from build123d import *

# Parameters (mm, degrees)
SKETCH_1_R          = 1.55
SKETCH_1_R_2        = 1.3
EXTRUDE_1_DEPTH     = 3
FILLET_1_R          = 1
SKETCH_2_W          = 7.568949752
SKETCH_2_H          = 24.928305666
CUT_EXTRUDE_1_DEPTH = 10


with BuildPart() as part:
    # 草图1 → 凸台-拉伸1 (new body)
    with BuildSketch(Plane(origin=(0, 0, 0), x_dir=(0, 0, -1), z_dir=(1, 0, 0))):
        with BuildLine():
            Line((-11, -27.75), (11, -27.75))
            Line((11, -27.75), (11, 19.65))
            Line((11, 19.65), (28.4, 19.65))
            Line((28.4, 19.65), (28.4, 25.85))
            ThreePointArc((28.4, 25.85), (29.45, 26.9), (30.5, 25.85))
            Line((30.5, 25.85), (43.6, 25.85))
            Line((43.6, 25.85), (43.6, 19.65))
            Line((43.6, 19.65), (45.6, 19.65))
            Line((45.6, 19.65), (45.6, 29.85))
            Line((45.6, 29.85), (19.913066695, 41.248539803))
            Line((19.913066695, 41.248539803), (-11, 27.75))
            Line((-11, 27.75), (-11, -27.75))
        make_face()
        with Locations((-8, -19.75)):
            Circle(SKETCH_1_R, mode=Mode.SUBTRACT)
        with Locations((0, -23.25)):
            Circle(SKETCH_1_R, mode=Mode.SUBTRACT)
        with Locations((0, -16.25)):
            Circle(SKETCH_1_R, mode=Mode.SUBTRACT)
        with Locations((8, -19.75)):
            Circle(SKETCH_1_R, mode=Mode.SUBTRACT)
        Polygon((5.344705464, -11.25), (-5.344705464, -11.25), (0, 0.202940281), align=None, mode=Mode.SUBTRACT)
        Polygon((-7, -7.702940281), (-7, 15.202940281), (-1.655294536, 3.75), align=None, mode=Mode.SUBTRACT)
        Polygon((7, 15.202940281), (7, -7.702940281), (1.655294536, 3.75), align=None, mode=Mode.SUBTRACT)
        with Locations((-6, 23.75)):
            Circle(SKETCH_1_R, mode=Mode.SUBTRACT)
        with BuildLine():
            Line((2, 16.7), (-2, 16.7))
            ThreePointArc((-2, 16.7), (-3.05, 15.65), (-4.1, 16.7))
            Line((-4.1, 16.7), (-4.1, 19.8))
            ThreePointArc((-4.1, 19.8), (-3.05, 20.85), (-2, 19.8))
            Line((-2, 19.8), (2, 19.8))
            ThreePointArc((2, 19.8), (3.05, 20.85), (4.1, 19.8))
            Line((4.1, 19.8), (4.1, 16.7))
            ThreePointArc((4.1, 16.7), (3.05, 15.65), (2, 16.7))
        make_face(mode=Mode.SUBTRACT)
        with Locations((6, 23.75)):
            Circle(SKETCH_1_R, mode=Mode.SUBTRACT)
        with Locations((15, 22.75)):
            Circle(SKETCH_1_R_2, mode=Mode.SUBTRACT)
        Polygon((11, 27.75), (-1.004338059, 27.75), (15.913066695, 35.137175905), (15.913066695, 27.75), align=None, mode=Mode.SUBTRACT)
        Polygon((23.913066695, 28.85), (23.913066695, 35.097405162), (37.991771729, 28.85), align=None, mode=Mode.SUBTRACT)
        with Locations((19.913066695, 36.248539803)):
            Circle(SKETCH_1_R_2, mode=Mode.SUBTRACT)
    extrude(amount=EXTRUDE_1_DEPTH)

    # 圆角1
    fillet_1_edges = [part.edges().sort_by_distance(p)[0] for p in [
        (1.5, 35.097405162, -23.913066695),
        (1.5, 28.85, -23.913066695),
        (1.5, 28.85, -37.991771729),
        (1.5, 35.137175905, -15.913066695),
        (1.5, 27.75, 1.004338059),
        (1.5, 27.75, -15.913066695),
        (1.5, 15.202940281, 7),
        (1.5, -7.702940281, 7),
        (1.5, 3.75, 1.655294536),
        (1.5, -7.702940281, -7),
        (1.5, 15.202940281, -7),
        (1.5, 3.75, -1.655294536),
        (1.5, -11.25, 5.344705464),
        (1.5, -11.25, -5.344705464),
        (1.5, 0.202940281, 0),
    ]]
    fillet(fillet_1_edges, radius=FILLET_1_R)

    # 草图2 → 切除-拉伸1 (cut)
    with BuildSketch(Plane(origin=(3, 0, 0), x_dir=(0, 0, -1), z_dir=(1, 0, 0))):
        with Locations((47.384474876, 32.114152833)):
            Rectangle(SKETCH_2_W, SKETCH_2_H)
    extrude(amount=-CUT_EXTRUDE_1_DEPTH, mode=Mode.SUBTRACT)


solid = part.part
Verification items for the finished model (mm, model axes). Coordinates: 2 decimals unless noted, no trailing zeros. Loops run counter-clockwise (first coordinate to the right, second up) from the corner with the lowest first, then second, coordinate; pieces in that order, holes last. Notation, with made-up numbers: (29, 63) -> (61, 63) arc R17 cw to (61, 70) -> close; hole circle Ø10 at (67.25, -8). An arc over 180 degrees is marked (long way). Answer as a JSON object with one key per item and string values. Group by question number.
Item 1: Sectioned sample at B-B on y = -19. Record the boundary of the cut face in (x, z), plus the area to 3 significant figures.
Item 2: Scan lines: probe 1 along Z at (x, y) = (2.7, 30); probe 2 along Y at (x, z) = (1.65, -5.5); probe 3 along Z at (x, y) = (1.4, 0.5). Record each from-to range of solid material in increasing order.
Item 3: Sectioned sample at A-A on z = 3.05. Record the boundary of the cut face in (x, y).
Item 4: Mould release check, pull along Z, two halves, no side actions. Record for faces 1 (the cylindrical face through (1.48, 20.85, 3.07)), 2 (the flat face through (1, 0, 11)): +Z half, -Z half, draft (parallel to the pull), parting line (faces both ways), or undercut.
Item 5: Sectioned sample at C-C on z = -27. Record the boundary of the cut face in (x, y), plus the area to 3 significant figures.
Item 6: Depth check by flat-ended pin: pin 1 (0.9 mm diameter, centred on x = 1, y = 32, fed in from +Z); pin 2 (0.9 mm diameter, centred on x = 1.5, z = 1, fed in from +Y); pin 3 (2.5 mm diameter, centred on y = -16.25, z = 0, fed in from +X); pin 4 (1 mm diameter, centred on x = 1, z = -18.5, fed in from +Y). Enter the tip coordinate at first touch or a pass-through.
Item 7: Sectioned sample at D-D on y = 5. Record the boundary of the cut face in (x, z).
Evaluation:
{
 "1": {"outline": "(0, -11) -> (3, -11) -> (3, -9.36) -> (0, -9.36) -> close; (0, -6.64) -> (3, -6.64) -> (3, 6.64) -> (0, 6.64) -> close; (0, 9.36) -> (3, 9.36) -> (3, 11) -> (0, 11) -> close", "area": "49.7 mm²"},
 "2": {"probe 1": "z = -43.6 to -34.26, -23.91 to -15.91, -4.15 to 5.85", "probe 2": "y = -27.75 to -4.06, 11.56 to 22.28, 25.22 to 27.75, 30.59 to 34.95", "probe 3": "z = -11 to -7, -3.17 to 3.17, 7 to 11"},
 "3": {"outline": "(0, -27.75) -> (3, -27.75) -> (3, -11.25) -> (0, -11.25) -> close; (0, -6.33) -> (3, -6.33) -> (3, 0.76) -> (0, 0.76) -> close; (0, 6.74) -> (3, 6.74) -> (3, 15.65) -> (0, 15.65) -> close; (0, 20.85) -> (3, 20.85) -> (3, 31.22) -> (0, 31.22) -> close"},
 "4": {"face 1": "undercut", "face 2": "+Z half"},
 "5": {"outline": "(0, 19.65) -> (3, 19.65) -> (3, 28.85) -> (0, 28.85) -> close; (0, 33.73) -> (3, 33.73) -> (3, 38.1) -> (0, 38.1) -> close", "area": "40.7 mm²"},
 "6": {"pin 1": "stops at z = 2.3", "pin 2": "stops at y = 32.31", "pin 3": "passes through", "pin 4": "stops at y = 40.85"},
 "7": {"outline": "(0, -11) -> (3, -11) -> (3, -7) -> (0, -7) -> close; (0, -2.24) -> (3, -2.24) -> (3, 2.24) -> (0, 2.24) -> close; (0, 7) -> (3, 7) -> (3, 11) -> (0, 11) -> close"}
}
